Check sheet for the drawn part. Datum: minimum x, y, z corner. Units: mm. Round coordinates to 2 decimals unless told otherwise and drop trailing zeros. Write each loop counter-clockwise with the first axis right and the second up, starting at its lowest first coordinate (ties: lowest second). Pieces come first, ordered by that corner, then holes. Notation, with made-up numbers: (37, 41) - (59, 41) arc R17 cw to (59, 61) - close; hole circle Ø5 at (9, -31). An arc over 180 degrees is marked (long way). Return JSON: item names as keys, results as strings. Group by question number.
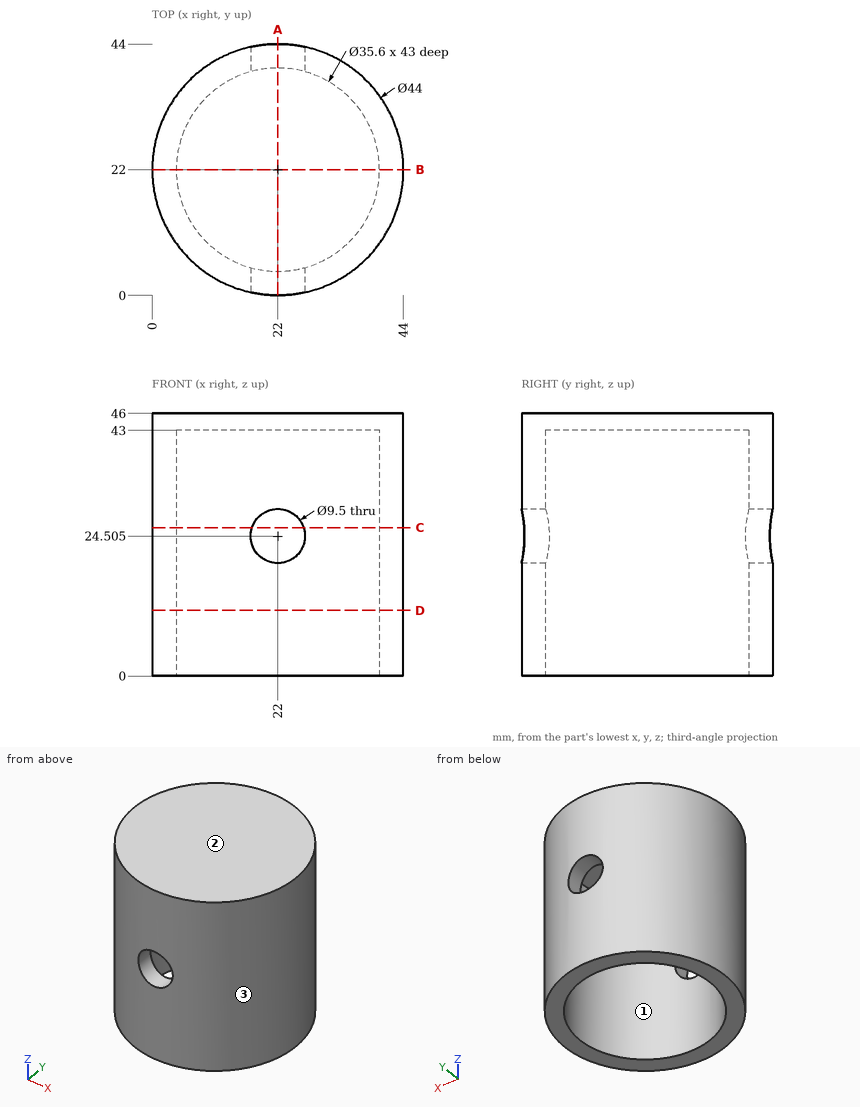
1. Section check B-B (y = 22). Enter the section's corners in (x, z), and give its area (3 significant figures).
2. Section check D-D (z = 11.5). Enter the section's corners in (x, y).
3. Section check A-A (x = 22). Enter the section's corners in (y, z) (3 decimals).
4. Mould release check, pull along X, two halves, no side actions. Record for the marked faces 1, 2 and 3: pulls with the +X half, pulls with the -X half, needs draft (parallel to the pull), parting line crosses it, or undercut.
5. Section check C-C (z = 26). Enter the section's corners in (x, y), and give its area (3 significant figures).
6. Depth check by flat-ended pin: pin 1 Ø1.5 at (y, z) = (27.5, 38) entering from +X; pin 2 Ø1.5 at (x, z) = (16, 30) entering from +Y; pin 3 Ø2 at (x, y) = (19, 35.5) entering from -Z. Enter the tip coordinate at first touch or a pass-through.
7. Material ranges on line 1 along Y through (x, z) = (22, 13); line 2 along Z through (x, y) = (36.5, 27.5); line 3 along X through (y, z) = (29, 37), recorded low to high.
Result sheet:
{
 "1": {"outline": "(0, 0) - (4.2, 0) - (4.2, 43) - (39.8, 43) - (39.8, 0) - (44, 0) - (44, 46) - (0, 46) - close", "area": "493 mm²"},
 "2": {"outline": "circle Ø44 at (22, 22); hole circle Ø35.6 at (22, 22)"},
 "3": {"outline": "(0, 0) - (4.2, 0) - (4.2, 19.755) - (0, 19.755) - close; (0, 29.255) - (4.2, 29.255) - (4.2, 43) - (39.8, 43) - (39.8, 29.255) - (44, 29.255) - (44, 46) - (0, 46) - close; (39.8, 0) - (44, 0) - (44, 19.755) - (39.8, 19.755) - close"},
 "4": {"face 1": "undercut", "face 2": "needs draft", "face 3": "parting line crosses it"},
 "5": {"outline": "(17.49, 0.47) - (17.49, 4.78) arc R17.8 cw to (17.49, 39.22) - (17.49, 43.53) arc R22 ccw to start; (26.51, 0.47) arc R22 ccw to (26.51, 43.53) - (26.51, 39.22) arc R17.8 cw to (26.51, 4.78) - close", "area": "449 mm²"},
 "6": {"pin 1": "stops at x = 43.48", "pin 2": "stops at y = 43.36", "pin 3": "stops at z = 43"},
 "7": {"line 1": "y = 0 to 4.2, 39.8 to 44", "line 2": "z = 43 to 46", "line 3": "x = 1.14 to 5.63, 38.37 to 42.86"}
}
